CAD build for the part. Positions are in the model's coordinates, mm. A direction names the side the tool comes from. Give positions to 0.01 mm unless a question says otherwise; leave off trailing zeros. Loops run counter-clockwise (first coordinate to the right, second up) from the corner with the lowest first, then second, coordinate; pieces in that order, holes last. Notation, with made-up numbers: M 69.5,42 L 73.5,42 A13 cw 73.5,65 Z; hole C 60.5,3 d11. An arc over 180 degrees is marked long. One line per question, with ' | ' between items.
```python
from build123d import *

# Parameters (mm, degrees)
F0_W      = 75.543475
F0_H      = 56.50536
F1_DEPTH  = 50.8
F2_W      = 37.771738
F2_H      = 56.50536
F3_DEPTH  = 38.1
F4_R      = 7.62
F5_R      = 5.08
F6_R      = 11.003795
F8_DEPTH  = 25.4
F7_R      = 10.16
F7_R_2    = 3.816716
F9_DEPTH  = 25.4
F7_R_3    = 4.942263
F10_DEPTH = 142.256165
F11_R     = 7.347925
F12_DEPTH = 124.534214


with BuildPart() as f1:
    # F0 (on Top) → F1 (new body)
    with BuildSketch(Plane.XY):
        with Locations((9.419816, -7.99929)):
            Rectangle(F0_W, F0_H)
    extrude(amount=F1_DEPTH)

    # F2 (on face) → F3 (join)
    with BuildSketch(Plane.XY.offset(50.8)):
        with Locations((-9.466053, -7.99929)):
            Rectangle(F2_W, F2_H)
    extrude(amount=F3_DEPTH)

    # F4
    f4_edges = [f1.edges().sort_by_distance(p)[0] for p in [
        (9.419816, -7.99929, 88.9),
    ]]
    fillet(f4_edges, radius=F4_R)

    # F5
    f5_edges = [f1.edges().sort_by_distance(p)[0] for p in [
        (47.191553, -7.99929, 50.8),
    ]]
    fillet(f5_edges, radius=F5_R)

    # F6 (on face) → F8 (join)
    with BuildSketch(Plane.XY.offset(88.9)):
        with Locations((-13.276053, -7.99929)):
            Circle(F6_R)
    extrude(amount=F8_DEPTH)

    # F7 (on face) → F9 (join)
    with BuildSketch(Plane.XY.offset(50.8)):
        with Locations((25.765684, -7.99929)):
            Circle(F7_R)
        with Locations((25.765684, -7.99929)):
            Circle(F7_R_2, mode=Mode.SUBTRACT)
    extrude(amount=F9_DEPTH)

    # F7 (on face) → F10 (cut)
    with BuildSketch(Plane.XY.offset(50.8)):
        with Locations((25.765684, 10.959573)):
            Circle(F7_R_3)
    extrude(amount=-F10_DEPTH, mode=Mode.SUBTRACT)

    # F11 (on face) → F12 (cut)
    with BuildSketch(Plane.XY.offset(114.3)):
        with Locations((-13.276053, -7.99929)):
            Circle(F11_R)
    extrude(amount=-F12_DEPTH, mode=Mode.SUBTRACT)


solid = f1.part
```
Item 1: Saw through at A-A on y = -10. Give the cut face in (x, z), and give its area (3 significant figures).
Conclusion:
outline: M -28.35,0 L -20.35,0 L -20.35,114.3 L -24.1,114.3 L -24.1,88.9 L -28.35,88.9 Z; M -6.21,0 L 47.19,0 L 47.19,45.72 A5.08 ccw 42.11,50.8 L 35.73,50.8 L 35.73,76.2 L 29.02,76.2 L 29.02,50.8 L 22.52,50.8 L 22.52,76.2 L 15.8,76.2 L 15.8,50.8 L 9.42,50.8 L 9.42,81.28 A7.62 ccw 1.8,88.9 L -2.46,88.9 L -2.46,114.3 L -6.21,114.3 Z | area: 4,530 mm²
Item 2: Saw through at D-D on x = 25. Give the cut face in (y, z), and give its area (3 significant figures).
Conclusion:
outline: M -36.25,0 L 6.08,0 L 6.08,50.8 L 2.13,50.8 L 2.13,76.2 L -4.26,76.2 L -4.26,50.8 L -11.74,50.8 L -11.74,76.2 L -18.13,76.2 L -18.13,50.8 L -36.25,50.8 Z; M 15.84,0 L 20.25,0 L 20.25,50.8 L 15.84,50.8 Z | area: 2,700 mm²
Item 3: Drop flat-ended pins along their axis: P1, Ø7, axis at x = 25.77, y = -8, coming from the +Z side; P2, Ø5, axis at y = -22.5, z = 49.5, coming from the +X side; P3, Ø22.5, axis at x = 30.5, y = -6.5, coming from the +Z side; P4, Ø6, axis at x = 25.77, y = 10.96, coming from the -Z side. Give the stop position or say it passes through.
Conclusion:
P1: z = 50.8 | P2: x = 47.03 | P3: z = 76.2 | P4: through
Item 4: Mould opens along X. For faces 4 (the flat face through (-28.352, -8, 70)), 5 (the cylindrical face through (18.28, -1.13, 63.32)), 6 (the flat face through (-6, -10, 114.3)) say: pulls with the +X half, pulls with the -X half, needs draft (parallel to the pull), parting line crosses it, or undercut.
Conclusion:
face 4: pulls with the -X half | face 5: undercut | face 6: needs draft
Item 5: Saw through at C-C on y = -31.5. Give the cut face in (x, z), and give its area (3 significant figures).
Conclusion:
outline: M -28.35,0 L 47.19,0 L 47.19,45.72 A5.08 ccw 42.11,50.8 L 9.42,50.8 L 9.42,81.28 A7.62 ccw 1.8,88.9 L -28.35,88.9 Z | area: 5,260 mm²
Item 6: Saw through at B-B on z = 55.5. Give the cut face in (x, y).
Conclusion:
outline: M -28.35,-36.25 L 9.42,-36.25 L 9.42,20.25 L -28.35,20.25 Z; C 25.77,-8 d20.32; hole C -13.28,-8 d14.7; hole C 25.77,-8 d7.63
Item 7: Drill centre lines: line 1 along X through (y, z) = (-14, 66); line 2 along X through (y, z) = (-9.5, 60); line 3 along Z through (x, y) = (-13.5, 7.5). Where is each one in solid material? Low to high. Write a range as [from, to].
Conclusion:
line 1: [-28.35, -17.52], [-9.04, 9.42], [17.57, 33.96] | line 2: [-28.35, -20.47], [-6.08, 9.42], [15.72, 22.26], [29.27, 35.81] | line 3: [0, 88.9]
Item 8: 3-axis set-ups, long thin cutter, end or side, ignore diameter. For faces 1 (the cylindrical face through (-22.01, -14.69, 101.42)), 2 (the flat face through (30, -8, 76.2)), 3 (the flat face through (0, 20.253, 34)): which of +Z, -Z, +X, -X, +Y, -Y reach the whole face in a straight line?
Conclusion:
face 1: +Z | face 2: +Z, +X, +Y, -Y | face 3: +Z, -Z, +X, -X, +Y
